Design review of the part shown in the three views and the two pictorial views. Dimensions are in mm from the part's minimum x, y and z. Give positions to 0.01 mm unless a question says otherwise; leave off trailing zeros. Order: outer loops, then holes, each group sorted by start corner. A loop starts at its lowest first (then second) coordinate and runs counter-clockwise, first axis right, second up. Notation, with made-up numbers: (44, -9) - (67, -9) arc R26 cw to (67, 18) - close; hole circle Ø11 at (68.25, -21). An arc over 180 degrees is marked (long way). Put each result on its own line as item: value.
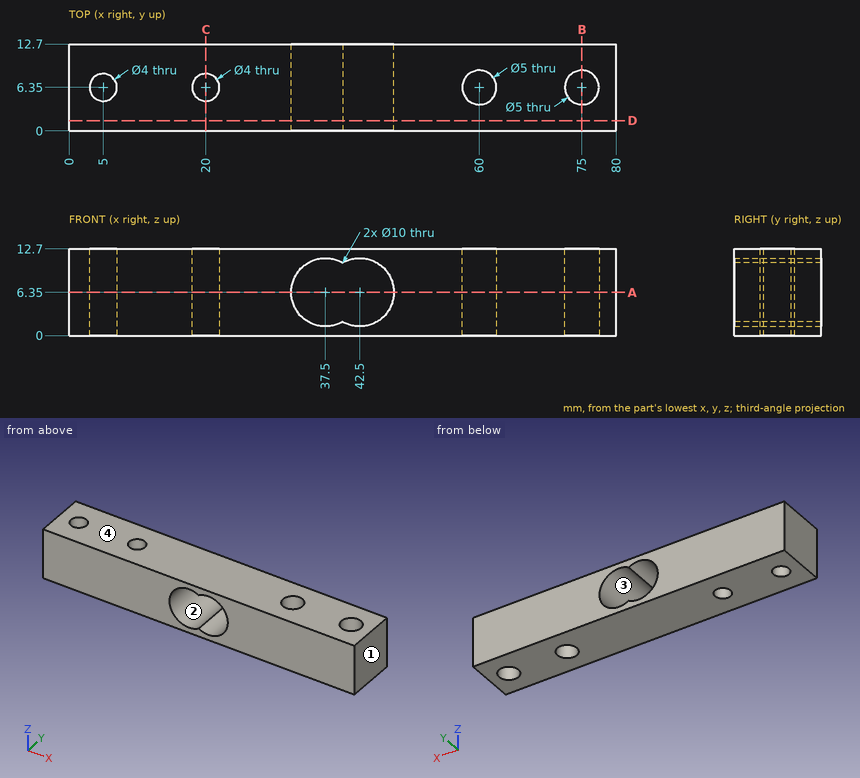
(1) Take a section at C-C, the plane x = 20. Write out the cut boundary in (y, z).
The answers:
outline: (0, 0) - (4.35, 0) - (4.35, 12.7) - (0, 12.7) - close; (8.35, 0) - (12.7, 0) - (12.7, 12.7) - (8.35, 12.7) - close
(2) Take a section at A-A, the plane z = 6.35. Write out the cut boundary in (x, y).
The answers:
outline: (0, 0) - (32.5, 0) - (32.5, 12.7) - (0, 12.7) - close; (47.5, 0) - (80, 0) - (80, 12.7) - (47.5, 12.7) - close; hole circle Ø4 at (5, 6.35); hole circle Ø4 at (20, 6.35); hole circle Ø5 at (60, 6.35); hole circle Ø5 at (75, 6.35)
(3) Take a section at D-D, the plane y = 1.5. Write out the cut boundary in (x, z).
The answers:
outline: (0, 0) - (80, 0) - (80, 12.7) - (0, 12.7) - close; hole (40, 2.02) arc R5 ccw (long way) to (40, 10.68) arc R5 ccw (long way) to start
(4) Clearance check with flat-ended pins moving along their axes: pin 1 Ø1.5 at (y, z) = (10, 9.5) entering from -X; pin 2 Ø4.5 at (x, y) = (60, 6.35) entering from +Z. State where each tip first meets the part, or that it passes through.
The answers:
pin 1: x = 0
pin 2: through
(5) Wall thickness on L1, parallel to X at y = 9, z = 6.5; L2, parallel to Y at x = 20, z = 10; L3, parallel to X at y = 6.75, z = 6.5: over which ranges is each line inside the solid? List them lowest first.
The answers:
L1: 0 to 32.5, 47.5 to 80
L2: 0 to 4.35, 8.35 to 12.7
L3: 0 to 3.04, 6.96 to 18.04, 21.96 to 32.5, 47.5 to 57.53, 62.47 to 72.53, 77.47 to 80
(6) Take a section at B-B, the plane x = 75. Write out the cut boundary in (y, z).
The answers:
outline: (0, 0) - (3.85, 0) - (3.85, 12.7) - (0, 12.7) - close; (8.85, 0) - (12.7, 0) - (12.7, 12.7) - (8.85, 12.7) - close
(7) The part is to be moulded in two halves that separate along X. For the marked faces 1, 2, 3 and 4, say which applies: pulls with the +X half, pulls with the -X half, needs draft (parallel to the pull), parting line crosses it, or undercut.
The answers:
face 1: pulls with the +X half
face 2: undercut
face 3: undercut
face 4: needs draft
